Design review of the part shown in the three views and the two pictorial views. Dimensions are in mm from the part's minimum x, y and z. A direction names the side the tool comes from. Give positions to 0.01 mm unless a question says otherwise; leave off trailing zeros. Order: outer loops, then holes, each group sorted by start corner. A loop starts at its lowest first (then second) coordinate and runs counter-clockwise, first axis right, second up. Notation, with made-up numbers: (81.25, -17) -> (115.25, -17) arc R33 cw to (115.25, 14) -> close; hole circle Ø2 at (6, 52). An arc over 180 degrees is marked (long way). Answer in a Markdown table with one row per item. Add a question column.
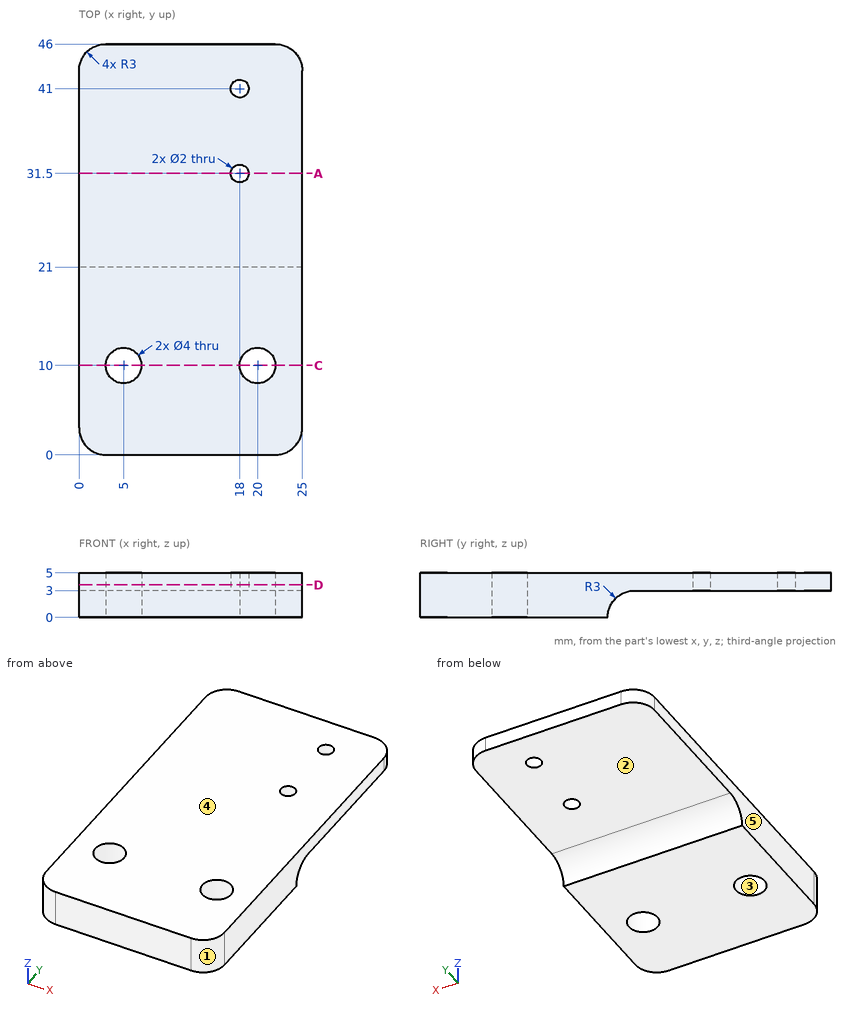
1) Add section A-A, the plane y = 31.5. Write out the cut boundary in (x, z).
2) Add section D-D, the plane z = 3.65. Write out the cut boundary in (x, y), and give its area (3 significant figures).
3) Add section C-C, the plane y = 10. Write out the cut boundary in (x, z).
4) Clearance check with flat-ended pins moving along their axes: P1, Ø1.6, axis at x = 18, y = 41, coming from the +Z side; P2, Ø6, axis at x = 12.5, y = 37, coming from the -Z side. State where each tip first meets the part, or that it passes through.
5) Mouldability with a two-part tool opening along X and no side actions: class the marked faces 3, 4 and 5 as +X half, -X half, draft (parallel to the pull), parting line (faces both ways), or undercut.
6) For L1, parallel to Y at x = 5, z = 3.3; L2, parallel to Z at x = 16, y = 25; L3, parallel to Y at x = 20, z = 2.6, list the stretches that pass through material, from the lowest coordinate up.
7) Machinability: for the marked faces 1 and 2, which of the approach directions +Z, -Z, +X, -X, +Y, -Y give a long, thin tool a straight path to every point of the face, cutting with its end or side? Answer none if there is none.
Verdict:
| question | item | result |
|---|---|---|
| 1 | outline | (0, 3) -> (17, 3) -> (17, 5) -> (0, 5) -> close; (19, 3) -> (25, 3) -> (25, 5) -> (19, 5) -> close |
| 2 | outline | (0, 3) arc R3 ccw to (3, 0) -> (22, 0) arc R3 ccw to (25, 3) -> (25, 43) arc R3 ccw to (22, 46) -> (3, 46) arc R3 ccw to (0, 43) -> close; hole circle Ø4 at (5, 10); hole circle Ø2 at (18, 31.5); hole circle Ø2 at (18, 41); hole circle Ø4 at (20, 10) |
| 2 | area | 1,110 mm2 |
| 3 | outline | (0, 0) -> (3, 0) -> (3, 5) -> (0, 5) -> close; (7, 0) -> (18, 0) -> (18, 5) -> (7, 5) -> close; (22, 0) -> (25, 0) -> (25, 5) -> (22, 5) -> close |
| 4 | P1 | passes through |
| 4 | P2 | stops at z = 3 |
| 5 | face 3 | undercut |
| 5 | face 4 | draft |
| 5 | face 5 | -X half |
| 6 | L1 | y = 0 to 8, 12 to 46 |
| 6 | L2 | z = 3 to 5 |
| 6 | L3 | y = 0 to 8, 12 to 22.5 |
| 7 | face 1 | +Z, -Z, +X, -Y |
| 7 | face 2 | -Z, +X, -X, +Y |
